Work out the finished part from the listing and answer in its coordinate system (mm). A direction names the side the tool comes from. Coordinates: 2 decimals unless noted, no trailing zeros. Loops run counter-clockwise (first coordinate to the right, second up) from the corner with the lowest first, then second, coordinate; pieces in that order, holes last. Notation, with made-up numbers: (27.25, 88.25) -> (48.25, 88.25) arc R32 ccw to (48.25, 126.25) -> close; hole circle Ø4 at (71.5, -10.5). An arc over 180 degrees is marked (long way). One line per question, with ' | ' between items.
```python
from build123d import *

# Parameters (mm, degrees)
F0_W      = 200
F0_H      = 1495.990298
F1_DEPTH  = 1300
F2_W      = 150
F2_H      = 300
F2_W_2    = 960
F2_H_2    = 280
F2_H_3    = 235.990298
F3_DEPTH  = 200
F4_W      = 160
F4_H      = 280
F4_H_2    = 300
F4_H_3    = 215.990298
F5_DEPTH  = 1150.001
F6_W      = 150
F6_H      = 20
F6_W_2    = 960
F7_DEPTH  = 1195.990298
F8_W      = 150
F8_H      = 404.009702
F8_H_2    = 400
F8_W_2    = 960
F8_H_3    = 20
F9_DEPTH  = 400.001
F10_W     = 360
F10_H     = 400
F10_H_2   = 404.009702
F11_DEPTH = 1150.001
F12_W     = 150
F12_H     = 20
F12_W_2   = 959.315732
F12_W_3   = 960.244403
F13_DEPTH = 884.010702


with BuildPart() as f1:
    # F0 (on Right) → F1 (new body)
    with BuildSketch(Plane.YZ):
        Polygon((-200, -1200), (200, -1200), (200, -295.990298), (0, -295.990298), (-200, -295.990298), align=None)
        with Locations((100, 452.004851)):
            Rectangle(F0_W, F0_H)
    extrude(amount=F1_DEPTH)

    # F2 (on face) → F3 (cut, through all)
    with BuildSketch(Plane.XZ):
        with Locations((75, 1050)):
            Rectangle(F2_W, F2_H)
        with Locations((650, 1050)):
            Rectangle(F2_W_2, F2_H)
        with Locations((1225, 1050)):
            Rectangle(F2_W, F2_H)
        with Locations((75, 730)):
            Rectangle(F2_W, F2_H)
        with Locations((650, 730)):
            Rectangle(F2_W_2, F2_H)
        with Locations((1225, 730)):
            Rectangle(F2_W, F2_H)
        with Locations((75, 410)):
            Rectangle(F2_W, F2_H)
        with Locations((650, 410)):
            Rectangle(F2_W_2, F2_H)
        with Locations((1225, 410)):
            Rectangle(F2_W, F2_H)
        with Locations((75, 100)):
            Rectangle(F2_W, F2_H_2)
        with Locations((650, 100)):
            Rectangle(F2_W_2, F2_H_2)
        with Locations((1225, 100)):
            Rectangle(F2_W, F2_H_2)
        with Locations((75, -177.995149)):
            Rectangle(F2_W, F2_H_3)
        with Locations((650, -177.995149)):
            Rectangle(F2_W_2, F2_H_3)
        with Locations((1225, -177.995149)):
            Rectangle(F2_W, F2_H_3)
    extrude(amount=-F3_DEPTH, mode=Mode.SUBTRACT)

    # F4 (on face) → F5 (cut, through all)
    with BuildSketch(Plane(origin=(150, 0, 0), x_dir=(0, -1, 0), z_dir=(-1, 0, 0))):
        with Locations((-100, 1040)):
            Rectangle(F4_W, F4_H)
        with Locations((-100, 730)):
            Rectangle(F4_W, F4_H_2)
        with Locations((-100, 410)):
            Rectangle(F4_W, F4_H_2)
        with Locations((-100, 100)):
            Rectangle(F4_W, F4_H)
        with Locations((-100, -167.995149)):
            Rectangle(F4_W, F4_H_3)
    extrude(amount=-F5_DEPTH, mode=Mode.SUBTRACT)

    # F6 (on face) → F7 (cut, through all)
    with BuildSketch(Plane.XY.offset(900)):
        with Locations((75, 190)):
            Rectangle(F6_W, F6_H)
        with Locations((75, 10)):
            Rectangle(F6_W, F6_H)
        with Locations((1225, 190)):
            Rectangle(F6_W, F6_H)
        with Locations((1225, 10)):
            Rectangle(F6_W, F6_H)
        with Locations((650, 190)):
            Rectangle(F6_W_2, F6_H)
        with Locations((650, 10)):
            Rectangle(F6_W_2, F6_H)
    extrude(amount=-F7_DEPTH, mode=Mode.SUBTRACT)

    # F8 (on face) → F9 (cut, through all)
    with BuildSketch(Plane.XZ.offset(200)):
        with Locations((1225, -957.995149)):
            Rectangle(F8_W, F8_H)
        with Locations((1225, -535.990298)):
            Rectangle(F8_W, F8_H_2)
        with Locations((650, -535.990298)):
            Rectangle(F8_W_2, F8_H_2)
        with Locations((650, -957.995149)):
            Rectangle(F8_W_2, F8_H)
        with Locations((75, -535.990298)):
            Rectangle(F8_W, F8_H_2)
        with Locations((75, -957.995149)):
            Rectangle(F8_W, F8_H)
        with Locations((75, -305.990298)):
            Rectangle(F8_W, F8_H_3)
        with Locations((650, -305.990298)):
            Rectangle(F8_W_2, F8_H_3)
        with Locations((1225, -305.990298)):
            Rectangle(F8_W, F8_H_3)
        with Locations((75, -1190)):
            Rectangle(F8_W, F8_H_3)
        with Locations((650, -1190)):
            Rectangle(F8_W_2, F8_H_3)
        with Locations((1225, -1190)):
            Rectangle(F8_W, F8_H_3)
    extrude(amount=-F9_DEPTH, mode=Mode.SUBTRACT)

    # F10 (on face) → F11 (cut, through all)
    with BuildSketch(Plane(origin=(150, 0, 0), x_dir=(0, -1, 0), z_dir=(-1, 0, 0))):
        with Locations((0, -535.990298)):
            Rectangle(F10_W, F10_H)
        with Locations((0, -957.995149)):
            Rectangle(F10_W, F10_H_2)
    extrude(amount=-F11_DEPTH, mode=Mode.SUBTRACT)

    # F12 (on face) → F13 (cut, through all)
    with BuildSketch(Plane.XY.offset(-315.990298)):
        with Locations((75, 190)):
            Rectangle(F12_W, F12_H)
        with Locations((75, -190)):
            Rectangle(F12_W, F12_H)
        with Locations((650.439762, 190)):
            Rectangle(F12_W_2, F12_H)
        with Locations((1225.097628, 190)):
            Rectangle(F12_W, F12_H)
        with Locations((1225, -190)):
            Rectangle(F12_W, F12_H)
        with Locations((649.975427, -190)):
            Rectangle(F12_W_3, F12_H)
    extrude(amount=-F13_DEPTH, mode=Mode.SUBTRACT)


solid = f1.part
```
1) For faces 1 (the face through (1224, 7, -1180)), 2 (the face through (1224, 7, -315.99)), determine the directions among +Z, -Z, +X, -X, +Y, -Y from which every point of the face is accessible in a straight line to the end or side of a thin tool.
Check values:
face 1: -Z, +X, +Y, -Y | face 2: +X, +Y, -Y
2) The mould has two halves that part along X. Classify faces 3 (the face through (1130, 192, 326)), 4 (the face through (643, 7, -1180)), 5 (the face through (74, -3, -315.99)): released by +X, released by -X, zero draft, split by the parting line, or undercut.
Check values:
face 3: undercut | face 4: undercut | face 5: zero draft
3) Find section A-A (y = -68). Write down the section's boundary in (x, z), plus the area to 3 significant figures.
Check values:
outline: (0, -1180) -> (150, -1180) -> (150, -1200) -> (170, -1200) -> (170, -1180) -> (1130, -1180) -> (1130, -1200) -> (1150, -1200) -> (1150, -1180) -> (1300, -1180) -> (1300, -1160) -> (0, -1160) -> close; (0, -755.99) -> (1300, -755.99) -> (1300, -735.99) -> (0, -735.99) -> close; (0, -335.99) -> (1300, -335.99) -> (1300, -315.99) -> (1150, -315.99) -> (1150, -295.99) -> (1130, -295.99) -> (1130, -315.99) -> (170, -315.99) -> (170, -295.99) -> (150, -295.99) -> (150, -315.99) -> (0, -315.99) -> close | area: 79,600 mm^2
4) Flat-ended cylindrical pins translate along their axes: pin 1 (6 mm diameter, centred on x = 1237, z = 566, fed in from +Y); pin 2 (10 mm diameter, centred on x = 1135.5, z = 432, fed in from -Y); pin 3 (5 mm diameter, centred on x = 808, y = -124, fed in from -Z). Find the tip coordinate at first contact, or state that the pin passes through.
Check values:
pin 1: stops at y = 180 | pin 2: stops at y = 0 | pin 3: stops at z = -1180
5) Find section B-B (x = 469). Write down the section's boundary in (y, z).
Check values:
outline: (-180, -1180) -> (180, -1180) -> (180, -1160) -> (-180, -1160) -> close; (-180, -755.99) -> (180, -755.99) -> (180, -735.99) -> (-180, -735.99) -> close; (-180, -335.99) -> (180, -335.99) -> (180, -315.99) -> (-180, -315.99) -> close; (20, -60) -> (180, -60) -> (180, -40) -> (20, -40) -> close; (20, 240) -> (180, 240) -> (180, 260) -> (20, 260) -> close; (20, 560) -> (180, 560) -> (180, 580) -> (20, 580) -> close; (20, 880) -> (180, 880) -> (180, 900) -> (20, 900) -> close
6) Find section C-C (z = -498.5). Write down the section's boundary in (x, y), plus the area to 3 significant figures.
Check values:
outline: (150, -200) -> (169.85, -200) -> (169.85, -180) -> (150, -180) -> close; (150, 180) -> (170, 180) -> (170, 200) -> (150, 200) -> close; (1130.1, -200) -> (1150, -200) -> (1150, -180) -> (1130.1, -180) -> close; (1130.1, 180) -> (1150, 180) -> (1150, 200) -> (1130.1, 200) -> close | area: 1,590 mm^2
7) Find the intervals of material crossed by line 1 along Z through (x, y) = (959, -95), in increasing order.
Check values:
line 1: z = -1180 to -1160, -755.99 to -735.99, -335.99 to -315.99
8) Find section D-D (z = 493). Write down the section's boundary in (x, y).
Check values:
outline: (150, 0) -> (170, 0) -> (170, 20) -> (150, 20) -> close; (150, 180) -> (170, 180) -> (170, 200) -> (150, 200) -> close; (1130, 0) -> (1150, 0) -> (1150, 20) -> (1130, 20) -> close; (1130, 180) -> (1150, 180) -> (1150, 200) -> (1130, 200) -> close
